```python
from build123d import *

# Parameters (mm, degrees)
SKETCH_1_R               = 3
EXTRUDE_1_DEPTH          = 15
M4X0_7_1_D               = 3.3
M4X0_7_1_DEPTH           = 8.5
M4X0_7_1_TIP             = 0.991420021
M4X0_7_1_ON_FACE_2_D     = 3.3
M4X0_7_1_ON_FACE_2_DEPTH = 8.5
M4X0_7_1_ON_FACE_2_TIP   = 0.991420021
M4X0_7_1_ON_FACE_3_D     = 3.3
M4X0_7_1_ON_FACE_3_DEPTH = 8.5
M4X0_7_1_ON_FACE_3_TIP   = 0.991420021


with BuildPart() as part:
    # ｽｹｯﾁ1 → ﾎﾞｽ - 押し出し1 (new body, symmetric)
    with BuildSketch(Plane.XY):
        Circle(SKETCH_1_R)
    extrude(amount=EXTRUDE_1_DEPTH, both=True)

    # M4x0.7 ねじ穴1
    with Locations(Plane.XY.offset(15)):
        with Locations((0, 0)):
            Hole(M4X0_7_1_D / 2, depth=M4X0_7_1_DEPTH)
            with Locations((0, 0, -(M4X0_7_1_DEPTH + M4X0_7_1_TIP / 2))):  # 118° drill point
                Cone(0, M4X0_7_1_D / 2, M4X0_7_1_TIP, mode=Mode.SUBTRACT)

    # M4x0.7 ねじ穴1 on face 2
    with Locations(Plane(origin=(0, 0, -15), x_dir=(-1, 0, 0), z_dir=(0, 0, -1))):
        with Locations((0, 0)):
            Hole(M4X0_7_1_ON_FACE_2_D / 2, depth=M4X0_7_1_ON_FACE_2_DEPTH)
            with Locations((0, 0, -(M4X0_7_1_ON_FACE_2_DEPTH + M4X0_7_1_ON_FACE_2_TIP / 2))):  # 118° drill point
                Cone(0, M4X0_7_1_ON_FACE_2_D / 2, M4X0_7_1_ON_FACE_2_TIP, mode=Mode.SUBTRACT)

    # M4x0.7 ねじ穴1 on face 3
    with Locations(Plane(origin=(8.523250275, 2.088443879, 0), x_dir=(1, 0, 0), z_dir=(0, 0, 1))):
        with Locations((0, 0)):
            Hole(M4X0_7_1_ON_FACE_3_D / 2, depth=M4X0_7_1_ON_FACE_3_DEPTH)
            with Locations((0, 0, -(M4X0_7_1_ON_FACE_3_DEPTH + M4X0_7_1_ON_FACE_3_TIP / 2))):  # 118° drill point
                Cone(0, M4X0_7_1_ON_FACE_3_D / 2, M4X0_7_1_ON_FACE_3_TIP, mode=Mode.SUBTRACT)


solid = part.part
```
Source: CAD feature listing. Evaluate the final solid. Frame: model axes, mm. A direction names the side the tool comes from. Coordinates: 2 decimals unless noted, no trailing zeros. Loops run counter-clockwise (first coordinate to the right, second up) from the corner with the lowest first, then second, coordinate; pieces in that order, holes last. Notation, with made-up numbers: M 37.25,84.25 L 79.25,84.25 A16 cw 79.25,91.25 Z; hole C 39.25,56 d6. An arc over 180 degrees is marked long. Use a Markdown table: item, result. Add a question column.
Q1. Material intervals for L1, parallel to Y at x = 0, z = -8.5; L2, parallel to Y at x = -0.75, z = 10.5, sorted ascending.
Q2. Draft query along Y for faces 4 (the flat face through (1.3, -1.3, 15)), 5 (the conical face through (0.1, -0.3, -5.7)), 6 (the cylindrical face through (-3, 0, 0)). Return one class per face: pulls with the +Y half, pulls with the -Y half, needs draft (parallel to the pull), parting line crosses it, or undercut.
Q3. First-contact query: pin 1 (2.5 mm diameter, centred on x = 0, y = 0, fed in from -Z). Flat tip, straight axial feed; report the tip coordinate or a pass-through.
Q4. Section query D-D, the plane y = 2.5. Return loops of the section in (x, z).
Q5. Section query A-A, the plane z = -7.75. Return loops of the section in (x, y), and give its area (3 significant figures).
Q6. Section query C-C, the plane z = 4.75. Return loops of the section in (x, y), and give its area (3 significant figures).
Q7. Section query B-B, the plane x = 2.4. Return loops of the section in (y, z), and give its area (3 significant figures).
Q8. Access query for faces 1 (the cylindrical face through (-1.216, 1.115, -10.69)), 2 (the cylindrical face through (1.216, 1.115, 10.69)), 3 (the flat face through (1.3, -1.3, -15)). Directions: +Z, -Z, +X, -X, +Y, -Y. A direction counts if a zero-diameter tool reaches every point of the face in a straight line with its end or side. Return the directions, or none.
Result:
| question | item | result |
|---|---|---|
| 1 | L1 | y = -3 to -1.65, 1.65 to 3 |
| 1 | L2 | y = -2.9 to -1.47, 1.47 to 2.9 |
| 2 | face 4 | needs draft |
| 2 | face 5 | undercut |
| 2 | face 6 | parting line crosses it |
| 3 | pin 1 | stops at z = -6.26 |
| 4 | outline | M -1.66,-15 L 1.66,-15 L 1.66,15 L -1.66,15 Z |
| 5 | outline | C 0,0 d6; hole C 0,0 d3.3 |
| 5 | area | 19.7 mm2 |
| 6 | outline | C 0,0 d6 |
| 6 | area | 28.3 mm2 |
| 7 | outline | M -1.8,-15 L 1.8,-15 L 1.8,15 L -1.8,15 Z |
| 7 | area | 108 mm2 |
| 8 | face 1 | -Z |
| 8 | face 2 | +Z |
| 8 | face 3 | -Z, +X, -X, +Y, -Y |
